```python
from build123d import *

# Parameters (mm, degrees)
CUT_EXTRUDE1_REACH = 23.81
SKETCH2_R          = 1.25


with BuildPart() as part:
    # Sketch1 → Revolve1 (revolve)
    with BuildSketch(Plane.XY, mode=Mode.PRIVATE) as revolve1_sk:
        Polygon((0, 0), (-6.2, 0), (-6.2, 12.6), (-12, 12.6), (-12, 13.7), (-2.35, 13.7), (-2.35, 17.1), (0, 17.1), align=None)
    revolve(revolve1_sk.sketch.rotate(Axis((0, 17.1, 0), (0, -1, 0)), 270), axis=Axis((0, 17.1, 0), (0, -1, 0)))

    # Sketch2 → Cut-Extrude1 (cut, up to next)
    with BuildSketch(Plane(origin=(0, 13.7, 0), x_dir=(1, 0, 0), z_dir=(0, 1, 0)), mode=Mode.PRIVATE) as cut_extrude1_sk1:
        with Locations(Location((0, 8.5, 0), (0, 0, 270))):
            Circle(SKETCH2_R)
    cut_extrude1_tool1 = extrude(cut_extrude1_sk1.sketch, amount=-CUT_EXTRUDE1_REACH, mode=Mode.PRIVATE) & part.part
    # Sketch2 → Cut-Extrude1 (cut, up to next)
    with BuildSketch(Plane(origin=(0, 13.7, 0), x_dir=(1, 0, 0), z_dir=(0, 1, 0)), mode=Mode.PRIVATE) as cut_extrude1_sk2:
        with Locations(Location((7.361215932, -4.25, 0), (0, 0, 270))):
            Circle(SKETCH2_R)
    cut_extrude1_tool2 = extrude(cut_extrude1_sk2.sketch, amount=-CUT_EXTRUDE1_REACH, mode=Mode.PRIVATE) & part.part
    # Sketch2 → Cut-Extrude1 (cut, up to next)
    with BuildSketch(Plane(origin=(0, 13.7, 0), x_dir=(1, 0, 0), z_dir=(0, 1, 0)), mode=Mode.PRIVATE) as cut_extrude1_sk3:
        with Locations(Location((-7.361215932, -4.25, 0), (0, 0, 270))):
            Circle(SKETCH2_R)
    cut_extrude1_tool3 = extrude(cut_extrude1_sk3.sketch, amount=-CUT_EXTRUDE1_REACH, mode=Mode.PRIVATE) & part.part
    add(cut_extrude1_tool1.solids().sort_by_distance((0, 13.7, -8.5))[0], mode=Mode.SUBTRACT)
    add(cut_extrude1_tool2.solids().sort_by_distance((7.361216, 13.7, 4.25))[0], mode=Mode.SUBTRACT)
    add(cut_extrude1_tool3.solids().sort_by_distance((-7.361216, 13.7, 4.25))[0], mode=Mode.SUBTRACT)


solid = part.part
```
Input: part model. Units: mm. Frame: model coordinates. A direction names the side the tool comes from. Give positions to 0.01 mm unless a question says otherwise; leave off trailing zeros. Write each loop counter-clockwise with the first axis right and the second up, starting at its lowest first coordinate (ties: lowest second). Pieces come first, ordered by that corner, then holes. Notation, with made-up numbers: (23, 34.5) - (29, 34.5) arc R22 cw to (29, 64.5) - close; hole circle Ø5 at (65.25, 17.5). An arc over 180 degrees is marked (long way). Write item = value, one per line. Start each with the question number.
1. Mould query, pull axis Z, two halves, no side actions, for faces 4 (the flat face through (0, 0, 0)), 5 (the cylindrical face through (-3.604, 13.158, 11.446)), 6 (the cylindrical face through (-8.58, 13.16, 3.98)), 7 (the cylindrical face through (8.415, 13.158, 4.922)). Classes: released by +Z, released by -Z, zero draft, split by the parting line, or undercut.
2. Section query D-D, the plane z = -8.5. Output: boundary loops of the cut face in (x, y), then the cut area to 3 significant figures.
3. Section query C-C, the plane z = 0. Output: boundary loops of the cut face in (x, y).
4. Section query A-A, the plane x = 0. Output: boundary loops of the cut face in (y, z), then the cut area to 3 significant figures.
5. Section query B-B, the plane z = 4.25. Output: boundary loops of the cut face in (x, y), then the cut area to 3 significant figures.
6. First-contact query: pin 1 Ø3 at (x, z) = (7.36, 4.25) entering from -Y; pin 2 Ø4 at (y, z) = (11.5, -3.5) entering from -X; pin 3 Ø1.5 at (x, y) = (-0.5, 5.5) entering from -Z; pin 4 Ø7 at (x, z) = (4, 4) entering from -Y. Flat tips, straight axial feed; report the tip coordinate or a pass-through.
7. Ray query, L1, parallel to X at y = 13.2, z = 4.25; L2, parallel to X at y = 12, z = -0.25; L3, parallel to Z at x = -1, y = 11.25. Return the intervals inside material, ascending.
8. Access query for faces 1 (the cylindrical face through (-1.9, 6.4, 5.9)), 2 (the flat face through (0, 17.1, 0)), 3 (the cylindrical face through (-0.71, 15.42, 2.24)). Directions: +Z, -Z, +X, -X, +Y, -Y. A direction counts if a zero-diameter tool reaches every point of the face in a straight line with its end or side. Return the directions, or none.
Check sheet entries:
q1.face_4 = zero draft
q1.face_5 = split by the parting line
q1.face_6 = undercut
q1.face_7 = undercut
q2.outline = (-8.47, 12.6) - (-1.25, 12.6) - (-1.25, 13.7) - (-8.47, 13.7) - close; (1.25, 12.6) - (8.47, 12.6) - (8.47, 13.7) - (1.25, 13.7) - close
q2.area = 15.9 mm2
q3.outline = (-12, 12.6) - (-6.2, 12.6) - (-6.2, 0) - (6.2, 0) - (6.2, 12.6) - (12, 12.6) - (12, 13.7) - (2.35, 13.7) - (2.35, 17.1) - (-2.35, 17.1) - (-2.35, 13.7) - (-12, 13.7) - close
q4.outline = (0, -6.2) - (12.6, -6.2) - (12.6, -7.25) - (13.7, -7.25) - (13.7, -2.35) - (17.1, -2.35) - (17.1, 2.35) - (13.7, 2.35) - (13.7, 12) - (12.6, 12) - (12.6, 6.2) - (0, 6.2) - close; (12.6, -12) - (13.7, -12) - (13.7, -9.75) - (12.6, -9.75) - close
q4.area = 196 mm2
q5.outline = (-11.22, 12.6) - (-8.61, 12.6) - (-8.61, 13.7) - (-11.22, 13.7) - close; (-6.11, 12.6) - (-4.51, 12.6) - (-4.51, 0) - (4.51, 0) - (4.51, 12.6) - (6.11, 12.6) - (6.11, 13.7) - (-6.11, 13.7) - close; (8.61, 12.6) - (11.22, 12.6) - (11.22, 13.7) - (8.61, 13.7) - close
q5.area = 133 mm2
q6.pin_1 = 12.6
q6.pin_2 = -11.86
q6.pin_3 = -6.2
q6.pin_4 = 0
q7.L1 = -11.22 to -8.61, -6.11 to 6.11, 8.61 to 11.22
q7.L2 = -6.19 to 6.19
q7.L3 = -6.12 to 6.12
q8.face_1 = -Y
q8.face_2 = +Z, -Z, +X, -X, +Y
q8.face_3 = +Y
